Autodesk Inventor part; units mm, degrees
ref_plane "YZ Plane" through (0, 0, 0) normal (1, 0, 0) x (0, 1, 0)
ref_plane "XZ Plane" through (0, 0, 0) normal (0, 1, 0) x (-1, 0, 0)
ref_plane "XY Plane" through (0, 0, 0) normal (0, 0, 1) x (1, 0, 0)
sketch "스케치1" plane through (0, 0, 0) normal (0, 0, 1) x (1, 0, 0)
  line L0 (-69.2252, 42.3816) -> (-64.2252, 42.3816)
  line L1 (-64.2252, 42.3816) -> (-64.2252, -37.6184)
  line L2 (-64.2252, -37.6184) -> (-69.2252, -37.6184)
  line L3 (-69.2252, -37.6184) -> (-69.2252, 42.3816)
  point P0 (0, 0)
  point P1 (-66.7252, 42.3816)
  dimension "d0" = 5
  dimension "d1" = 80
extrude "돌출1" add sketch "스케치1" along normal blind 1
sketch "스케치2" plane through (0, 0, 1) normal (0, 0, 1) x (1, 0, 0)
  line L0 (-64.2252, 42.3816) -> (-69.2252, 42.3816)
  line L1 (-69.2252, 42.3816) -> (-64.2252, 42.3816)
  line L2 (-64.2252, 42.3816) -> (-64.2252, 37.3816)
  line L3 (-64.2252, 37.3816) -> (-69.2252, 37.3816)
  line L4 (-69.2252, 37.3816) -> (-69.2252, 42.3816)
  point P0 (0, 0)
  dimension "d7" = 5
  dimension "d8" = 5
extrude "돌출2" add sketch "스케치2" along normal blind 5
properties part number "display lock pin_3D 인쇄"
Design review of the part built by this model. Coordinates are the model's own, in mm. A direction names the side the tool comes from. Give positions to 0.01 mm unless a question says otherwise; leave off trailing zeros. Loops run counter-clockwise (first coordinate to the right, second up) from the corner with the lowest first, then second, coordinate; pieces in that order, holes last. Notation, with made-up numbers: M -33,-17.5 L -29,-17.5 A31 ccw -29,8.5 Z; hole C 73.5,62.25 d3. An arc over 180 degrees is marked long. Write item = value, one per line.
Q1. We need section A-A (x = -66.45). Give the boundary of the cut face in (y, z), plus the area to 3 significant figures.
Output values:
outline = M -37.62,0 L 42.38,0 L 42.38,6 L 37.38,6 L 37.38,1 L -37.62,1 Z
area = 105 mm^2
Q2. To check wall thickness, follow line 1 (Y direction, x = -66.75, z = 5.1); line 2 (Z direction, x = -65.15, y = 13.5). State the ranges of each line that lie inside material, in increasing order. Write a range as [from, to].
Output values:
line_1 = [37.38, 42.38]
line_2 = [0, 1]
Q3. We need section B-B (y = -16). Give the boundary of the cut face in (x, z), plus the area to 3 significant figures.
Output values:
outline = M -69.23,0 L -64.23,0 L -64.23,1 L -69.23,1 Z
area = 5.00 mm^2
Q4. Insertion check: pin 1 (2 mm diameter, centred on y = -20, z = 3, fed in from +X); pin 2 (1.5 mm diameter, centred on x = -68, y = -18.5, fed in from +Z); pin 3 (1.5 mm diameter, centred on x = -68, z = 4, fed in from -Y). Each pin has a flat end and moves straight along its axis. Give the tip position at first contact, or say it passes through.
Output values:
pin_1 = through
pin_2 = 1
pin_3 = 37.38
Q5. We need section C-C (z = 4). Give the boundary of the cut face in (x, y), plus the area to 3 significant figures.
Output values:
outline = M -69.23,37.38 L -64.23,37.38 L -64.23,42.38 L -69.23,42.38 Z
area = 25.0 mm^2
Q6. For faces 1 (the flat face through (-69.225, 11.1, 0.5)), 2 (the flat face through (-67, 0, 1)), list the 3-axis set-ups (+Z, -Z, +X, -X, +Y, -Y) from which the entire face can be reached by the end or side of a thin tool; tool diameter is ignored.
Output values:
face_1 = +Z, -Z, -X, +Y, -Y
face_2 = +Z, +X, -X, -Y
